Design review of the part shown in the three views and the two pictorial views. Dimensions are in mm from the part's minimum x, y and z. Coordinates: 2 decimals unless noted, no trailing zeros. Write each loop counter-clockwise with the first axis right and the second up, starting at its lowest first coordinate (ties: lowest second). Pieces come first, ordered by that corner, then holes. Notation, with made-up numbers: (0, 5.5) - (24, 5.5) arc R18 cw to (24, 27.5) - close; hole circle Ø5 at (15.25, 2). An arc over 180 degrees is marked (long way). Return JSON: item names as keys, results as strings. Group by question number.
(1) We need section C-C on x = 5. State the section outline as (y, z) points, then the cut area to 3 significant figures.
(2) To check wall thickness, follow L1, parallel to Y at x = 40, z = 7.5; L2, parallel to X at y = 94.16, z = 3.5; L3, parallel to Y at x = 60.5, z = 9. State the ranges of each line that lie inside material, in increasing order. Write a range as from..to.
(3) Draft analysis for pull direction X (two halves, no side actions). For the marked faces 1, 2, 3 and 4, state which applies: released by +X, released by -X, zero draft, split by the parting line, or undercut.
(4) We need section B-B on y = 79.5. State the section outline as (x, z) points.
(5) We need section D-D on y = 94.16. State the section outline as (x, z) points.
(6) We need section A-A on x = 40. State the section outline as (y, z) points, then the cut area to 3 significant figures.
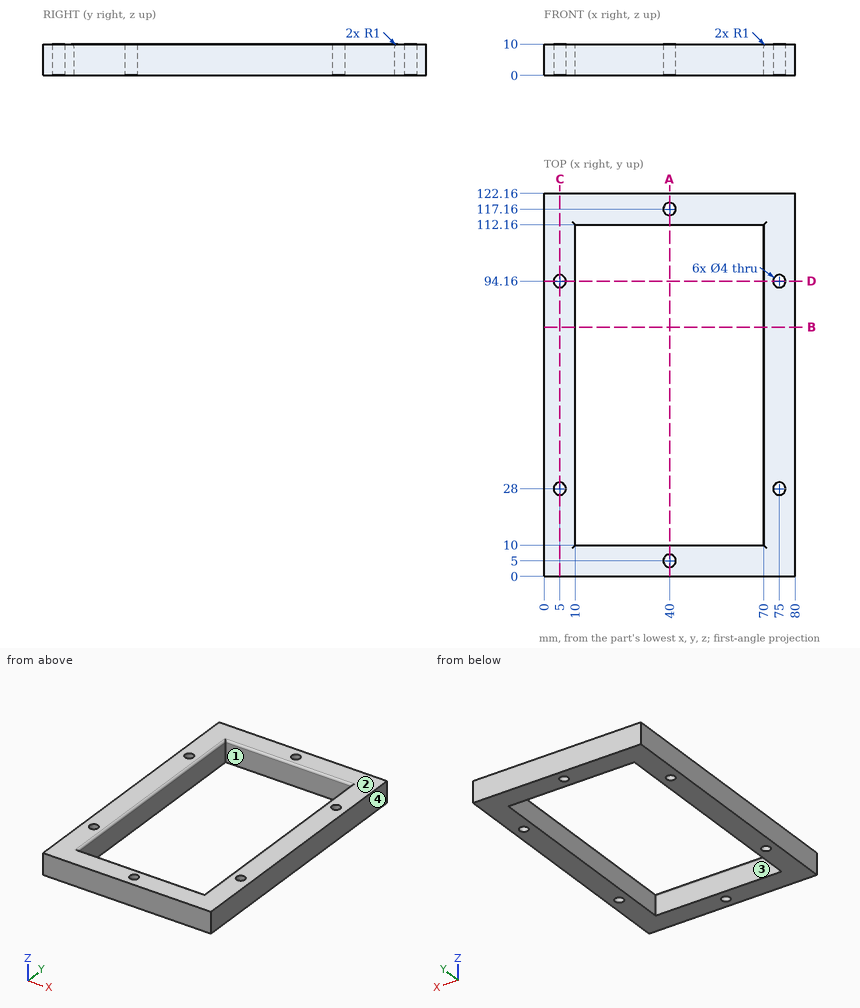
Ans:
{
 "1": {"outline": "(0, 0) - (26, 0) - (26, 10) - (0, 10) - close; (30, 0) - (92.16, 0) - (92.16, 10) - (30, 10) - close; (96.16, 0) - (122.16, 0) - (122.16, 10) - (96.16, 10) - close", "area": "1,140 mm²"},
 "2": {"L1": "0..3, 7..10, 112.16..115.16, 119.16..122.16", "L2": "0..3, 7..10, 70..73, 77..80", "L3": "0..10, 112.16..122.16"},
 "3": {"face 1": "undercut", "face 2": "zero draft", "face 3": "undercut", "face 4": "released by +X"},
 "4": {"outline": "(0, 0) - (10, 0) - (10, 9) arc R1 ccw to (9, 10) - (0, 10) - close; (70, 0) - (80, 0) - (80, 10) - (71, 10) arc R1 ccw to (70, 9) - close"},
 "5": {"outline": "(0, 0) - (3, 0) - (3, 10) - (0, 10) - close; (7, 0) - (10, 0) - (10, 9) arc R1 ccw to (9, 10) - (7, 10) - close; (70, 0) - (73, 0) - (73, 10) - (71, 10) arc R1 ccw to (70, 9) - close; (77, 0) - (80, 0) - (80, 10) - (77, 10) - close"},
 "6": {"outline": "(0, 0) - (3, 0) - (3, 10) - (0, 10) - close; (7, 0) - (10, 0) - (10, 9) arc R1 ccw to (9, 10) - (7, 10) - close; (112.16, 0) - (115.16, 0) - (115.16, 10) - (113.16, 10) arc R1 ccw to (112.16, 9) - close; (119.16, 0) - (122.16, 0) - (122.16, 10) - (119.16, 10) - close", "area": "120 mm²"}
}
